Read the model definition and answer for the solid it produces. Units are mm, in the model's axes. A direction names the side the tool comes from. Coordinates: 2 decimals unless noted, no trailing zeros. Loops run counter-clockwise (first coordinate to the right, second up) from the corner with the lowest first, then second, coordinate; pieces in that order, holes last. Notation, with made-up numbers: (15.25, -30) -> (61.25, -30) arc R18 cw to (61.25, -13) -> close; hole circle Ø3 at (57, 0). An arc over 180 degrees is marked (long way). Answer as CSV lines item,"result".
```python
from build123d import *

# Parameters (mm, degrees)
F0_R     = 1.9381566851
F0_R_2   = 2.0917368597
F1_DEPTH = 1


# Not quite as in the source:
# - a feature names something its author has since deleted; it is built from what else it names


with BuildPart() as f1:
    # F0 (on Top) → F1 (new body)
    with BuildSketch(Plane.XY):
        with BuildLine():
            Line((3.1245559464, 26.2624721611), (-1.08e-08, 26.2624721611))
            Line((-1.08e-08, 26.2624721611), (-3.124555968, 26.2624721611))
            Line((-3.124555968, 26.2624721611), (-3.124555968, 28.8313598976))
            Line((-3.124555968, 28.8313598976), (-3.124555968, 38.4353779081))
            Line((-3.124555968, 38.4353779081), (-3.124555968, 40.0192436593))
            Line((-3.124555968, 40.0192436593), (-7.0351105106, 40.0192436593))
            Line((-7.0351105106, 40.0192436593), (-22.9566536529, 7.5476728616))
            add(Edge.make_bspline(
                [(-22.9566536529, 7.5476728616), (-25.3127067939, 4.1178797379), (-27.103694983, 0.0661364302), (-27.9845091561, -4.0443276364)],
                knots=[0, 0, 0, 0, 12.635418731, 12.635418731, 12.635418731, 12.635418731], degree=3))
            Line((-27.9845091561, -4.0443276364), (-24.3406626732, -5.7663835679))
            Line((-24.3406626732, -5.7663835679), (-24.3406626732, -6.0127781864))
            Line((-24.3406626732, -6.0127781864), (-27.9845091561, -6.501597853))
            Line((-27.9845091561, -6.501597853), (-27.9845091561, -13.1704901951))
            Line((-27.9845091561, -13.1704901951), (-24.3406626732, -13.83388813))
            Line((-24.3406626732, -13.83388813), (-24.3406626732, -14.0802827486))
            Line((-24.3406626732, -14.0802827486), (-28.1370117447, -15.4628727929))
            ThreePointArc((-28.1370117447, -15.4628727929), (-18.7026452725, -33.0246464869), (-0.0200514, -39.9804967013))
            ThreePointArc((-0.0200514, -39.9804967013), (-0.0100256971, -39.9804519319), (-1.08e-08, -39.9804036034))
            ThreePointArc((-1.08e-08, -39.9804036034), (18.6950876239, -33.0312342783), (28.1370117231, -15.4628727929))
            Line((28.1370117231, -15.4628727929), (24.3406626516, -14.0802827486))
            Line((24.3406626516, -14.0802827486), (24.3406626516, -13.8338881301))
            Line((24.3406626516, -13.8338881301), (27.9845091345, -13.1704901951))
            Line((27.9845091345, -13.1704901951), (27.9845091345, -6.501597853))
            Line((27.9845091345, -6.501597853), (24.3406626516, -6.0127781865))
            Line((24.3406626516, -6.0127781865), (24.3406626516, -5.7663835679))
            Line((24.3406626516, -5.7663835679), (27.9845091345, -4.0443276364))
            add(Edge.make_bspline(
                [(26.0221502825, 2.0106991689), (26.8752917045, 0.0540824437), (27.5438186439, -1.9877730517), (27.9845091345, -4.0443276364)],
                knots=[6.3136438899, 6.3136438899, 6.3136438899, 6.3136438899, 12.635418731, 12.635418731, 12.635418731, 12.635418731], degree=3))
            add(Edge.make_bspline(
                [(22.9566536312, 7.5476728616), (24.1339221361, 5.8338798437), (25.1701061555, 3.9647993294), (26.0221502825, 2.0106991689)],
                knots=[0, 0, 0, 0, 6.3136438899, 6.3136438899, 6.3136438899, 6.3136438899], degree=3))
            Line((22.9566536312, 7.5476728616), (21.8193497392, 9.8671744024))
            Line((21.8193497392, 9.8671744024), (7.035110489, 40.0192436593))
            Line((7.035110489, 40.0192436593), (3.1245559464, 40.0192436593))
            Line((3.1245559464, 40.0192436593), (3.1245559464, 38.4353779081))
            Line((3.1245559464, 38.4353779081), (3.1245559464, 28.8313598976))
            Line((3.1245559464, 28.8313598976), (3.1245559464, 26.2624721611))
        make_face()
        with Locations((-6.7846685267, -26.966459513)):
            Circle(F0_R, mode=Mode.SUBTRACT)
        with Locations((-1.08e-08, -28.2356044358)):
            Circle(F0_R, mode=Mode.SUBTRACT)
        with Locations((-4.7346279243, -21.1471724542)):
            Circle(F0_R, mode=Mode.SUBTRACT)
        with Locations((-1.08e-08, -22.3102177961)):
            Circle(F0_R, mode=Mode.SUBTRACT)
        with Locations((6.784668505, -26.966459513)):
            Circle(F0_R, mode=Mode.SUBTRACT)
        with Locations((4.7346279027, -21.1471724542)):
            Circle(F0_R, mode=Mode.SUBTRACT)
        with Locations((-12.4288502443, 18.366707164)):
            Circle(F0_R_2, mode=Mode.SUBTRACT)
        with Locations((-8.3437176479, 27.1654560115)):
            Circle(F0_R_2, mode=Mode.SUBTRACT)
        with Locations((12.4288502227, 18.366707164)):
            Circle(F0_R_2, mode=Mode.SUBTRACT)
        with Locations((8.3437176263, 27.1654560115)):
            Circle(F0_R_2, mode=Mode.SUBTRACT)
        with BuildLine():
            Line((21.8193497392, 14.0026268734), (21.8193497392, 9.8671744024))
            Line((21.8193497392, 9.8671744024), (22.9566536312, 7.5476728616))
            add(Edge.make_bspline(
                [(22.9566536312, 7.5476728616), (24.1339221361, 5.8338798437), (25.1701061555, 3.9647993294), (26.0221502825, 2.0106991689)],
                knots=[0, 0, 0, 0, 6.3136438899, 6.3136438899, 6.3136438899, 6.3136438899], degree=3))
            Line((26.0221502825, 2.0106991689), (28.4720553036, 3.5966005617))
            Line((28.4720553036, 3.5966005617), (28.4720553036, 14.0026268734))
            Line((28.4720553036, 14.0026268734), (26.9772648538, 17.9472138793))
            Line((26.9772648538, 17.9472138793), (23.1570666214, 17.9472138793))
            Line((23.1570666214, 17.9472138793), (21.8193497392, 14.0026268734))
        make_face()
        Polygon((23.0341097003, 14.6254569428), (23.103940836, 15.2695124223), (23.7673383417, 15.2695124223), (23.6930889239, 14.6254569428), align=None, mode=Mode.SUBTRACT)
        Polygon((27.2249650291, 14.6254569428), (26.5659858056, 14.6254569428), (26.4917363877, 15.2695124223), (27.1551338935, 15.2695124223), align=None, mode=Mode.SUBTRACT)
        Polygon((23.1912288972, 15.8630787924), (23.4530965144, 17.4342844956), (23.9942903911, 17.4342844956), (23.8371694774, 15.8630787924), align=None, mode=Mode.SUBTRACT)
        Polygon((24.238699366, 14.6254569428), (24.5689903023, 17.4904718284), (25.6900844272, 17.4904718284), (26.0203753635, 14.6254569428), align=None, mode=Mode.SUBTRACT)
        Polygon((27.0678458323, 15.8630787924), (26.4219052521, 15.8630787924), (26.2647843384, 17.4342844956), (26.8059782151, 17.4342844956), align=None, mode=Mode.SUBTRACT)
        Polygon((-3.124555968, 38.4353779081), (-3.124555968, 28.8313598976), (-2.8081914709, 29.1106844403), (-2.8081914709, 38.1560533654), align=None)
        Polygon((2.8081914492, 29.1106844403), (3.1245559464, 28.8313598976), (3.1245559464, 38.4353779081), (2.8081914492, 38.1560533654), align=None)
    extrude(amount=F1_DEPTH)


solid = f1.part
```
Q1. For faces 1 (the face through (14.53, 24.73, 0.49)), 2 (the face through (27.23, 2.793, 0.493)), 3 (the face through (7.679, -28.686, 0.493)), 4 (the face through (-26.188, -4.893, 0.493)), determine the directions among +Z, -Z, +X, -X, +Y, -Y from which every point of the face is accessible in a straight line to the end or side of a thin tool.
Results:
face 1,"+Z, -Z, +Y"
face 2,"+Z, -Z, +X"
face 3,"+Z, -Z"
face 4,"+Z, -Z, -X"
Q2. Given pin 1 Ø0.5 at (y, z) = (27, 0.5) entering from -X; pin 2 Ø0.5 at (y, z) = (12.5, 0.5) entering from -X; pin 3 Ø0.5 at (y, z) = (39, 0.5) entering from -X, each flat-ended and moving along its own axis, determine where each tip first touches the part or whether it passes through.
Results:
pin 1,"stops at x = -13.54"
pin 2,"stops at x = -20.65"
pin 3,"stops at x = -7.66"
Q3. A cutting plane is placed at A-A, the plane z = 0.45. Give the number of separate pieces and of enclosed holes in the cut face, and give its area (3 significant figures).
Results:
separate pieces,"1"
enclosed holes,"15"
area,"3,110 mm²"
Q4. A cutting plane is placed at B-B, the plane y = -31. Write down the section's boundary in (x, z).
Results:
outline,"(-20.8, 0) -> (20.8, 0) -> (20.8, 1) -> (-20.8, 1) -> close"
Q5. For a pull along X with two mould halves and no side action, classify faces 5 (the face through (26.137, -4.917, 0.493)), 6 (the face through (0, -8, 1)), 7 (the face through (-12.7, 20.44, 0.49)) as pulls with the +X half, pulls with the -X half, needs draft (parallel to the pull), parting line crosses it, or undercut.
Results:
face 5,"pulls with the +X half"
face 6,"needs draft"
face 7,"undercut"
Q6. Find the intervals of material crossed by probe 1 along X at (y, z) = (-9, 0.6); probe 2 along Y at (x, z) = (8.5, 0.7); probe 3 along X at (y, z) = (15.5, 0.8), in increasing order. Write a range as [from, to].
Results:
probe 1,"x = [-27.98, 27.98]"
probe 2,"y = [-38.72, -27.87], [-26.06, 25.08], [29.25, 37.03]"
probe 3,"x = [-19.06, 19.06], [22.33, 24.34], [25.92, 27.9]"
